Geometry: final body of the model. Coordinates: model frame, mm. A direction names the side the tool comes from. Give positions to 0.01 mm unless a question says otherwise; leave off trailing zeros. Write each loop counter-clockwise with the first axis right and the second up, starting at its lowest first coordinate (ties: lowest second). Pieces come first, ordered by that corner, then holes. Notation, with made-up numbers: (50, 86) - (57, 86) arc R22 ccw to (57, 101) - close; hole circle Ø2 at (-39, -27.5). An arc over 180 degrees is marked (long way). Use CSV: the item, a comma, the result in double quotes. Start each with the question number.
(1) Draft query along Z for faces 1 (the flat face through (0.2, 0, 2.4)), 2 (the cylindrical face through (-6.2, 15.21, 2.69)), 3 (the flat face through (0.361, 14.79, 2.235)). Return one class per face: released by +Z, released by -Z, zero draft, split by the parting line, or undercut.
(2) First-contact query: pin 1 Ø3 at (y, z) = (11, 0) entering from +X; pin 2 Ø1 at (x, y) = (-5, 10) entering from +Z; pin 3 Ø6 at (x, y) = (-1.5, 7.5) entering from +Z. Flat tips, straight axial feed; report the tip coordinate or a pass-through.
(3) Section A-A on y = 26.25. Output: boundary loops of the cut face in (x, z), and give its area (3 significant figures).
(4) Reachability of faces 4 (the flat face through (0.21, 14.79, -2.24)), 5 (the flat face through (-6, 15, 0)), 6 (the flat face through (0.115, 14.79, -2.745)) from +Z, -Z, +X, -X, +Y, -Y: full face, straight path, thin tool, end or side. Return the list, or none.
(5) Section C-C on z = -0.5. Output: boundary loops of the cut face in (x, y).
(6) Line query: probe 1 along X at (y, z) = (14, 0.5); probe 2 along Z at (x, y) = (-5.25, 25.5); probe 3 along Z at (x, y) = (0, 13.5). Output: solid intervals per line, ascending. Write a range as [from, to].
(7) Section B-B on x = 0.75. Output: boundary loops of the cut face in (y, z), and give its area (3 significant figures).
from build123d import *

# Parameters (mm, degrees)
BOSS_EXTRUDE1_DEPTH = 30
FILLET1_R           = 1


with BuildPart() as part:
    # Sketch1 → Boss-Extrude1 (new body)
    with BuildSketch(Plane(origin=(0, 0, 0), x_dir=(1, 0, 0), z_dir=(0, 1, 0))):
        Polygon((-6, -2.5), (-6, 2.5), (6, 2), (7, 3.09567943), (7, 3.59567943), (6, 2.5), (-6.5, 3.020833333), (-6.5, -3.020833333), (6, -2.5), (7, -3.59567943), (7, -3.09567943), (6, -2), align=None)
    extrude(amount=BOSS_EXTRUDE1_DEPTH)

    # Fillet1
    fillet1_edges = [part.edges().sort_by_distance(p)[0] for p in [
        (-6.5, 15, 3.020833333),
        (-6.5, 15, -3.020833333),
        (6, 15, -2.5),
        (7, 15, -3.09567943),
        (6, 15, -2),
        (-6, 15, -2.5),
        (-6, 15, 2.5),
        (6, 15, 2),
        (7, 15, 3.09567943),
        (6, 15, 2.5),
    ]]
    fillet(fillet1_edges, radius=FILLET1_R)


solid = part.part
Check values:
1,face 1,"zero draft"
1,face 2,"released by +Z"
1,face 3,"undercut"
2,pin 1,"stops at x = -6"
2,pin 2,"stops at z = 2.98"
2,pin 3,"stops at z = 2.94"
3,outline,"(-6.5, -1.98) arc R1 ccw to (-5.46, -2.98) - (5.53, -2.52) arc R1 cw to (6.31, -2.84) - (7, -3.6) - (7, -3.48) arc R1 ccw to (6.74, -2.81) - (6.31, -2.34) arc R1 ccw to (5.53, -2.02) - (-4.96, -2.46) arc R1 cw to (-6, -1.46) - (-6, 1.46) arc R1 cw to (-4.96, 2.46) - (5.53, 2.02) arc R1 ccw to (6.31, 2.34) - (6.74, 2.81) arc R1 ccw to (7, 3.48) - (7, 3.6) - (6.31, 2.84) arc R1 cw to (5.53, 2.52) - (-5.46, 2.98) arc R1 ccw to (-6.5, 1.98) - close"
3,area,"16.0 mm²"
4,face 4,"+Y, -Y"
4,face 5,"+X, +Y, -Y"
4,face 6,"-Z, +Y, -Y"
5,outline,"(-6.5, 0) - (-6, 0) - (-6, 30) - (-6.5, 30) - close"
6,probe 1,"x = [-6.5, -6]"
6,probe 2,"z = [-2.97, -2.43], [2.43, 2.97]"
6,probe 3,"z = [-2.75, -2.25], [2.25, 2.75]"
7,outline,"(0, -2.72) - (30, -2.72) - (30, -2.22) - (0, -2.22) - close; (0, 2.22) - (30, 2.22) - (30, 2.72) - (0, 2.72) - close"
7,area,"30.0 mm²"
